from build123d import *

# Parameters (mm, degrees)
SKETCH1_R               = 30
BOSS_EXTRUDE1_DEPTH     = 4
BOSS_EXTRUDE2_DEPTH     = 10
SKETCH3_W               = 22
SKETCH3_H               = 16
BOSS_EXTRUDE3_DEPTH     = 6
SKETCH5_R               = 10.5
BOSS_EXTRUDE4_DEPTH     = 4
SKETCH7_R               = 6.5
CUT_EXTRUDE3_DEPTH      = 9
CUT_EXTRUDE3_DEPTH_BACK = 9


with BuildPart() as part:
    # Sketch1 → Boss-Extrude1 (new body)
    with BuildSketch(Plane(origin=(0, 0, 0), x_dir=(0, 1, 0), z_dir=(0, 0, 1))):
        Circle(SKETCH1_R)
    extrude(amount=BOSS_EXTRUDE1_DEPTH)

    # Sketch2 → Boss-Extrude2 (add)
    with BuildSketch(Plane.XY.offset(4)):
        with BuildLine():
            Line((9.72022002, -20.845079102), (13.946402637, -29.908156972))
            Line((13.946402637, -29.908156972), (33, -21.023318607))
            Line((33, -21.023318607), (33, 95.492736163))
            Line((33, 95.492736163), (-2, 120))
            Line((-2, 120), (-2, 106))
            Line((-2, 106), (18.356238926, 88.919087425))
            ThreePointArc((18.356238926, 88.919087425), (21.782001231, 84.454547067), (23, 78.960509665))
            Line((23, 78.960509665), (23, 52.006989528))
            ThreePointArc((23, 52.006989528), (20.964088796, 45.02209462), (15.494037403, 40.224988297))
            Line((15.494037403, 40.224988297), (0, 33))
            Line((0, 33), (0, 21.96622081))
            Line((0, 21.96622081), (4.505962597, 24.067385677))
            ThreePointArc((4.505962597, 24.067385677), (16.984894909, 23.249473241), (23, 12.285384445))
            Line((23, 12.285384445), (23, -6.370702608))
            ThreePointArc((23, -6.370702608), (20.964088796, -13.355597517), (15.494037403, -18.15270384))
            Line((15.494037403, -18.15270384), (9.72022002, -20.845079102))
        make_face()
    extrude(amount=BOSS_EXTRUDE2_DEPTH)

    # Sketch3 → Boss-Extrude3 (add)
    with BuildSketch(Plane(origin=(-2, 0, 0), x_dir=(0, -1, 0), z_dir=(-1, 0, 0))):
        with Locations((-113, 8)):
            Rectangle(SKETCH3_W, SKETCH3_H)
    extrude(amount=BOSS_EXTRUDE3_DEPTH)

    # Sketch5 → Boss-Extrude4 (add)
    with BuildSketch(Plane.XY.offset(4)):
        Circle(SKETCH5_R)
    extrude(amount=BOSS_EXTRUDE4_DEPTH)

    # Sketch7 → Cut-Extrude3 (cut, two sides)
    with BuildSketch(Plane.XY.offset(8)) as cut_extrude3_sk:
        Circle(SKETCH7_R)
    extrude(amount=CUT_EXTRUDE3_DEPTH, mode=Mode.SUBTRACT)
    extrude(cut_extrude3_sk.sketch, amount=-CUT_EXTRUDE3_DEPTH_BACK, mode=Mode.SUBTRACT)


solid = part.part
Work out the finished part from the listing and answer in its coordinate system (mm). A direction names the side the tool comes from. Give positions to 0.01 mm unless a question says otherwise; leave off trailing zeros. Loops run counter-clockwise (first coordinate to the right, second up) from the corner with the lowest first, then second, coordinate; pieces in that order, holes last. Notation, with made-up numbers: M 34.5,-7.75 L 38.5,-7.75 A22 ccw 38.5,16.25 Z; hole C -2,-17 d7. An arc over 180 degrees is marked long. Use CSV: the item, a comma, the result in double quotes.
1) Consider L1, parallel to Y at x = 0, z = 1.75; L2, parallel to Z at x = -7.5, y = -21; L3, parallel to X at y = 105, z = 6. Determine where each line is inside the solid, lowest interval first.
Answer:
L1,"-30 to -6.5, 6.5 to 30"
L2,"0 to 4"
L3,"-8 to -2, -0.81 to 19.42"
2) Which of the six approach directions +Z, -Z, +X, -X, +Y, -Y give full straight-line access (tool end or side, diameter ignored) to faces 1 (the flat face through (33, 36, 9)), 2 (the cylindrical face through (21, -13.3, 8.9)), 3 (the flat face through (7.855, 36.663, 8.93)), 4 (the cylindrical face through (-1.32, -29.97, 1.97))?
Answer:
face 1,"+Z, -Z, +X, +Y, -Y"
face 2,"+Z"
face 3,"+Z, -Z, -X"
face 4,"-Z"
3) Find section C-C on y = 17. Write down the section's boundary in (x, z), plus the area to 3 significant figures.
Answer:
outline,"M -24.72,0 L 24.72,0 L 24.72,4 L 33,4 L 33,14 L 22.11,14 L 22.11,4 L -24.72,4 Z"
area,"307 mm^2"
4) Find section A-A on y = 0. Write down the section's boundary in (x, z).
Answer:
outline,"M -30,0 L -6.5,0 L -6.5,8 L -10.5,8 L -10.5,4 L -30,4 Z; M 6.5,0 L 30,0 L 30,4 L 33,4 L 33,14 L 23,14 L 23,4 L 10.5,4 L 10.5,8 L 6.5,8 Z"
5) Find section B-B on z = 10.75. Write down the section's boundary in (x, y), plus the area to 3 significant figures.
Answer:
outline,"M -8,102 L -2,102 L -2,106 L 18.36,88.92 A13 cw 23,78.96 L 23,52.01 A13 cw 15.49,40.22 L 0,33 L 0,21.97 L 4.51,24.07 A13 cw 23,12.29 L 23,-6.37 A13 cw 15.49,-18.15 L 9.72,-20.85 L 13.95,-29.91 L 33,-21.02 L 33,95.49 L -2,120 L -2,124 L -8,124 Z"
area,"2,250 mm^2"
6) Determine the mould class of faces 5 (the flat face through (23, 46, 14)), 6 (the cylindrical face through (-5.158, -3.955, 4.056)), 7 (the flat face through (-10, -7, 4)), 8 (the flat face through (11.804, -25.313, 8.93)) for opening direction X: released by +X, released by -X, zero draft, split by the parting line, or undercut.
Answer:
face 5,"zero draft"
face 6,"undercut"
face 7,"undercut"
face 8,"released by -X"
7) Find section D-D on x = -24. Write down the section's boundary in (y, z).
Answer:
outline,"M -18,0 L 18,0 L 18,4 L -18,4 Z"
8) Given P1, Ø5, axis at y = 113.5, z = 11.5, coming from the -X side; P2, Ø5, axis at x = -5, z = 12, coming from the -Y side; P3, Ø6, axis at y = 102, z = 12, coming from the +X side, each flat-ended and moving along its own axis, determine where each tip first touches the part or whether it passes through.
Answer:
P1,"x = -8"
P2,"y = 102"
P3,"x = 27.99"
